Design review of the part built by this model. Coordinates are the model's own, in mm. Coordinates: 2 decimals unless noted, no trailing zeros. Use a Markdown table: item, result. Add a question column.
Q1. Add section C-C (z = -36). Count the separate pieces of the cut face and the enclosed holes in it, then the cut area to 3 significant figures.
Q2. Wall thickness on probe 1 along X at (y, z) = (-0.5, -18.5) (3 decimals); probe 2 along Z at (x, y) = (2.5, -3); probe 3 along Z at (x, y) = (-8.5, -5.5): over which ranges is each line inside the solid? List them lowest first.
Q3. Insertion check: pin 1 (3 mm diameter, centred on y = -1.5, z = 36, fed in from -X); pin 2 (1 mm diameter, centred on x = -4.5, y = -4.5, fed in from -Z); pin 3 (3 mm diameter, centred on x = 22.5, y = -3, fed in from -Z); pin 4 (3 mm diameter, centred on y = -4.5, z = -23, fed in from -X). Each pin has a flat end and moves straight along its axis. Give the tip position at first contact, or say it passes through.
from build123d import *

# Parameters (mm, degrees)
F0_W      = 88.9
F0_H      = 127
F1_DEPTH  = 6.35
F2_R      = 6.34999
F3_W      = 38.1
F3_H      = 38.1
F4_DEPTH  = 6.351
F5_W      = 20.32
F5_H      = 38.1
F5_W_2    = 10.16
F6_DEPTH  = 6.351
F7_W      = 4.318
F7_H      = 3.048
F8_DEPTH  = 3.048
F9_W      = 4.318
F9_H      = 3.048
F10_DEPTH = 3.048


# Not quite as in the source:
# - a fillet or chamfer is up to 0.001 mm smaller than in the source, because OpenCascade refuses the exact size


with BuildPart() as f1:
    # F0 (on Front) → F1 (new body)
    with BuildSketch(Plane.XZ):
        Rectangle(F0_W, F0_H)
    extrude(amount=F1_DEPTH)

    # F2 (radius 6.35 in the source; OpenCascade refuses exactly that, so slightly less here)
    f2_edges = [f1.edges().sort_by_distance(p)[0] for p in [
        (-44.45, -6.35, 0),
        (0, -6.35, 63.5),
        (44.45, -6.35, 0),
        (0, -6.35, -63.5),
    ]]
    fillet(f2_edges, radius=F2_R)

    # F3 (on face) → F4 (cut, through all)
    with BuildSketch(Plane.XZ.offset(6.35)):
        with Locations((0, 25.4)):
            Rectangle(F3_W, F3_H)
    extrude(amount=-F4_DEPTH, mode=Mode.SUBTRACT)

    # F5 (on face) → F6 (cut, through all)
    with BuildSketch(Plane.XZ.offset(6.35)):
        with Locations((0, -25.4)):
            Rectangle(F5_W, F5_H)
        with Locations((-24.765, -25.4)):
            Rectangle(F5_W_2, F5_H)
        with Locations((24.765, -25.4)):
            Rectangle(F5_W_2, F5_H)
    extrude(amount=-F6_DEPTH, mode=Mode.SUBTRACT)

    # F7 (on face) → F8 (cut)
    with BuildSketch(Plane.YZ.offset(-19.05)):
        with Locations((-2.159, 35.56)):
            Rectangle(F7_W, F7_H)
        with Locations((-2.159, 15.24)):
            Rectangle(F7_W, F7_H)
    extrude(amount=-F8_DEPTH, mode=Mode.SUBTRACT)

    # F9 (on face) → F10 (cut)
    with BuildSketch(Plane(origin=(19.05, 0, 0), x_dir=(0, -1, 0), z_dir=(-1, 0, 0))):
        with Locations((2.159, 15.24)):
            Rectangle(F9_W, F9_H)
        with Locations((2.159, 35.56)):
            Rectangle(F9_W, F9_H)
    extrude(amount=-F10_DEPTH, mode=Mode.SUBTRACT)


solid = f1.part
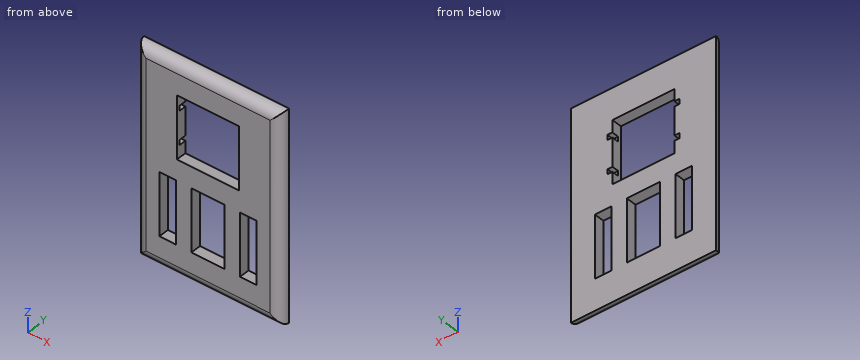
Established:
| question | item | result |
|---|---|---|
| 1 | separate pieces | 4 |
| 1 | enclosed holes | 0 |
| 1 | area | 289 mm^2 |
| 2 | probe 1 | -44.43 to -29.845, -19.685 to -10.16, 10.16 to 19.685, 29.845 to 44.43 |
| 2 | probe 2 | -62.75 to -44.45, -6.35 to 6.35, 44.45 to 62.75 |
| 2 | probe 3 | -60.32 to -44.45, -6.35 to 6.35, 44.45 to 60.32 |
| 3 | pin 1 | x = -44.45 |
| 3 | pin 2 | z = -62.08 |
| 3 | pin 3 | z = -63.32 |
| 3 | pin 4 | x = -43.7 |
